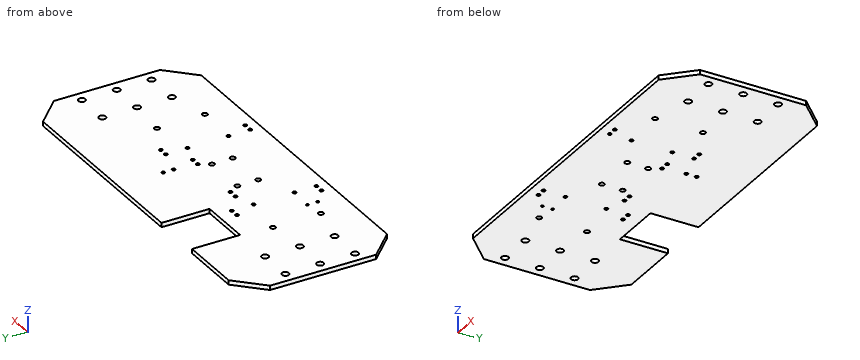
```python
from build123d import *

# Parameters (mm, degrees)
SKETCH_1_W          = 425
SKETCH_1_H          = 182
EXTRUDE_1_DEPTH     = 5
SKETCH_2_R          = 3
SKETCH_2_R_2        = 4
SKETCH_2_R_3        = 2
SKETCH_2_R_4        = 1.5
CUT_EXTRUDE_2_DEPTH = 232.219051983
SKETCH_3_W          = 60
SKETCH_3_H          = 55.25
CUT_EXTRUDE_3_DEPTH = 10
CHAMFER_1_SIZE      = 30


with BuildPart() as part:
    # 草图1 → 凸台-拉伸1 (new body)
    with BuildSketch(Plane.XY):
        Rectangle(SKETCH_1_W, SKETCH_1_H)
    extrude(amount=EXTRUDE_1_DEPTH)

    # 草图2 → 切除-拉伸2 (cut, through all)
    with BuildSketch(Plane.XY):
        with Locations((-25, -11)):
            Circle(SKETCH_2_R)
        with Locations((-25, -35)):
            Circle(SKETCH_2_R)
        with Locations(Location((25, -35, 0), (0, 0, 180))):
            Circle(SKETCH_2_R)
        with Locations(Location((25, -11, 0), (0, 0, 180))):
            Circle(SKETCH_2_R)
        with Locations((-200, 36)):
            Circle(SKETCH_2_R_2)
        with Locations((-160, 36)):
            Circle(SKETCH_2_R_2)
        with Locations((-200, -4)):
            Circle(SKETCH_2_R_2)
        with Locations((-160, -4)):
            Circle(SKETCH_2_R_2)
        with Locations(Location((160, -4, 0), (0, 0, 180))):
            Circle(SKETCH_2_R_2)
        with Locations(Location((200, -4, 0), (0, 0, 180))):
            Circle(SKETCH_2_R_2)
        with Locations(Location((160, 36, 0), (0, 0, 180))):
            Circle(SKETCH_2_R_2)
        with Locations(Location((200, 36, 0), (0, 0, 180))):
            Circle(SKETCH_2_R_2)
        with Locations((-200, -44)):
            Circle(SKETCH_2_R_2)
        with Locations((-160, -44)):
            Circle(SKETCH_2_R_2)
        with Locations(Location((160, -44, 0), (0, 0, 180))):
            Circle(SKETCH_2_R_2)
        with Locations(Location((200, -44, 0), (0, 0, 180))):
            Circle(SKETCH_2_R_2)
        with Locations((-32, 1)):
            Circle(SKETCH_2_R_3)
        with Locations((-42, 1)):
            Circle(SKETCH_2_R_3)
        with Locations(Location((32, 1, 0), (0, 0, 180))):
            Circle(SKETCH_2_R_3)
        with Locations(Location((42, 1, 0), (0, 0, 180))):
            Circle(SKETCH_2_R_3)
        with Locations((35, 39)):
            Circle(SKETCH_2_R_3)
        with Locations((35, 27)):
            Circle(SKETCH_2_R_3)
        with Locations((-75, -78.5)):
            Circle(SKETCH_2_R_3)
        with Locations((-65, -78.5)):
            Circle(SKETCH_2_R_3)
        with Locations((-65, -53.5)):
            Circle(SKETCH_2_R_3)
        with Locations((-65, -6.5)):
            Circle(SKETCH_2_R_3)
        with Locations((-65, 18.5)):
            Circle(SKETCH_2_R_3)
        with Locations((-75, 18.5)):
            Circle(SKETCH_2_R_3)
        with Locations(Location((75, -78.5, 0), (0, 0, 180))):
            Circle(SKETCH_2_R_3)
        with Locations(Location((65, -78.5, 0), (0, 0, 180))):
            Circle(SKETCH_2_R_3)
        with Locations(Location((65, -53.5, 0), (0, 0, 180))):
            Circle(SKETCH_2_R_3)
        with Locations(Location((65, -6.5, 0), (0, 0, 180))):
            Circle(SKETCH_2_R_3)
        with Locations(Location((65, 18.5, 0), (0, 0, 180))):
            Circle(SKETCH_2_R_3)
        with Locations(Location((75, 18.5, 0), (0, 0, 180))):
            Circle(SKETCH_2_R_3)
        with Locations((-114, -55)):
            Circle(SKETCH_2_R)
        with Locations((-114, 0)):
            Circle(SKETCH_2_R)
        with Locations(Location((114, 0, 0), (0, 0, 180))):
            Circle(SKETCH_2_R)
        with Locations(Location((114, -55, 0), (0, 0, 180))):
            Circle(SKETCH_2_R)
        with Locations((-92.5, -52)):
            Circle(SKETCH_2_R_4)
        with Locations((-92.5, -64)):
            Circle(SKETCH_2_R_4)
    extrude(amount=CUT_EXTRUDE_2_DEPTH, mode=Mode.SUBTRACT)

    # 草图3 → 切除-拉伸3 (cut)
    with BuildSketch(Plane.XY.offset(5)):
        with Locations((-80.5, 63.375)):
            Rectangle(SKETCH_3_W, SKETCH_3_H)
    extrude(amount=-CUT_EXTRUDE_3_DEPTH, mode=Mode.SUBTRACT)

    # 倒角1
    chamfer_1_edges = [part.edges().sort_by_distance(p)[0] for p in [
        (-212.5, 91, 2.5),
        (212.5, 91, 2.5),
        (212.5, -91, 2.5),
        (-212.5, -91, 2.5),
    ]]
    chamfer(chamfer_1_edges, length=CHAMFER_1_SIZE)


solid = part.part
```
The model under review builds one solid part; all positions refer to its coordinate system, in mm. Give positions to 0.01 mm unless a question says otherwise; leave off trailing zeros. Write each loop counter-clockwise with the first axis right and the second up, starting at its lowest first coordinate (ties: lowest second). Pieces come first, ordered by that corner, then holes. Notation, with made-up numbers: M -25,59 L 27,59 A25 cw 27,92 Z; hole C 5,53.25 d7. An arc over 180 degrees is marked long. Write each question's results on one line, items separated by ' | '. Start each with the question number.
1. We need section A-A (y = 68). Write out the cut boundary in (x, z).
2. We need section B-B (z = 1.2). Count the separate pieces of the cut face and the enclosed holes in it, and give its area (3 significant figures).
3. For probe 1 along Y at (x, z) = (-25, 3.3); probe 2 along Y at (x, z) = (35, 3.5); probe 3 along Y at (x, z) = (-160, 3.9), list the stretches that pass through material, from the lowest coordinate up. Write a range as [from, to].
Results found:
1) outline: M -205.5,0 L -110.5,0 L -110.5,5 L -205.5,5 Z; M -50.5,0 L 205.5,0 L 205.5,5 L -50.5,5 Z
2) separate pieces: 1 | enclosed holes: 40 | area: 71,200 mm^2
3) probe 1: y = [-91, -38], [-32, -14], [-8, 91] | probe 2: y = [-91, 25], [29, 37], [41, 91] | probe 3: y = [-91, -48], [-40, -8], [0, 32], [40, 91]
